The listing builds one solid part. Answer for the finished solid, in the listing's coordinates (mm). A direction names the side the tool comes from. Coordinates: 2 decimals unless noted, no trailing zeros. Order: outer loops, then holes, each group sorted by start corner. A loop starts at its lowest first (then second) coordinate and runs counter-clockwise, first axis right, second up. Notation, with made-up numbers: (18, 7) - (32, 7) arc R16 cw to (32, 34) - close; hole circle Ø2 at (55.25, 57.5). An arc over 180 degrees is marked (long way). Use a Markdown table: item, result. Add a question column.
Item 1: The part is cut by section B-B, the plane y = 6. Give the vertices of the cut face in (x, z).
Item 2: The part is cut by section D-D, the plane x = -0.75. Give the vertices of the cut face in (y, z).
Item 3: The part is cut by section C-C, the plane z = -0.15. Give the vertices of the cut face in (x, y), then the cut area to 3 significant figures.
Item 4: The part is cut by section A-A, the plane x = 5. Give the vertices of the cut face in (y, z).
Item 5: Find the intervals of material crossed by line 1 along Z through (x, y) = (1.75, 9); line 2 along X through (y, z) = (-16, 0.9); line 3 along X through (y, z) = (-6.5, -2.3), in increasing order.
Item 6: For faces 1 (the flat face through (-1.5, 0, 0)), 2 (the flat face through (3, 0, -1.5)), determine the directions among +Z, -Z, +X, -X, +Y, -Y from which every point of the face is accessible in a straight line to the end or side of a thin tool.
Item 7: A flat-ended cylindrical pin translates along its axis: P1, Ø0.9, axis at y = 4, z = 0.5, coming from the +X side. Find the tip coordinate at first contact, or state that the pin passes through.
Item 8: The mould has two halves that part along Z. Classify faces 3 (the flat face through (-0.3, -24.1, 0)), 4 (the flat face through (3, 0, 3)), 5 (the flat face through (3, 0, -3)), 6 (the flat face through (3, 0, 1.5)): released by +Z, released by -Z, zero draft, split by the parting line, or undercut.
from build123d import *

# Parameters (mm, degrees)
F1_DEPTH = 24.1
F2_R     = 1.5


with BuildPart() as f1:
    # F0 (on Front) → F1 (new body, symmetric)
    with BuildSketch(Plane.XZ):
        Polygon((0, 1.5), (6, 1.5), (6, 3), (-1.5, 3), (-1.5, -3), (6, -3), (6, -1.5), (0, -1.5), align=None)
    extrude(amount=F1_DEPTH, both=True)

    # F2
    f2_edges = [f1.edges().sort_by_distance(p)[0] for p in [
        (-1.5, 0, 3),
        (-1.5, 0, -3),
    ]]
    fillet(f2_edges, radius=F2_R)


solid = f1.part
Solution:
| question | item | result |
|---|---|---|
| 1 | outline | (-1.5, -1.5) arc R1.5 ccw to (0, -3) - (6, -3) - (6, -1.5) - (0, -1.5) - (0, 1.5) - (6, 1.5) - (6, 3) - (0, 3) arc R1.5 ccw to (-1.5, 1.5) - close |
| 2 | outline | (-24.1, -2.8) - (24.1, -2.8) - (24.1, 2.8) - (-24.1, 2.8) - close |
| 3 | outline | (-1.5, -24.1) - (0, -24.1) - (0, 24.1) - (-1.5, 24.1) - close |
| 3 | area | 72.3 mm2 |
| 4 | outline | (-24.1, -3) - (24.1, -3) - (24.1, -1.5) - (-24.1, -1.5) - close; (-24.1, 1.5) - (24.1, 1.5) - (24.1, 3) - (-24.1, 3) - close |
| 5 | line 1 | z = -3 to -1.5, 1.5 to 3 |
| 5 | line 2 | x = -1.5 to 0 |
| 5 | line 3 | x = -1.27 to 6 |
| 6 | face 1 | +Z, -Z, -X, +Y, -Y |
| 6 | face 2 | +X, +Y, -Y |
| 7 | P1 | stops at x = 0 |
| 8 | face 3 | zero draft |
| 8 | face 4 | released by +Z |
| 8 | face 5 | released by -Z |
| 8 | face 6 | undercut |
